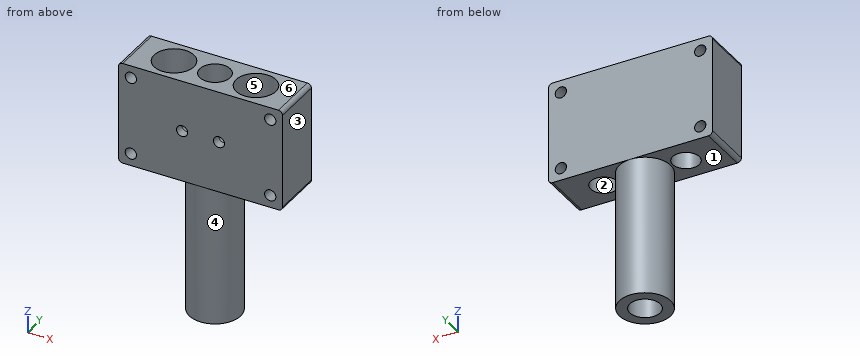
```python
from build123d import *
from OCP.BRepFilletAPI import BRepFilletAPI_MakeChamfer

# Parameters (mm, degrees)
SKETCH1_W            = 80
SKETCH1_H            = 50
BOSS_EXTRUDE1_DEPTH  = 25
M5_CLEARANCE_HOLE1_D = 5.5
SKETCH5_R            = 12.5
SKETCH5_R_2          = 6.985
BOSS_EXTRUDE2_DEPTH  = 68
SKETCH4_R            = 9.7
CUT_EXTRUDE2_DEPTH   = 29
SKETCH4_4_R          = 7.4
CUT_EXTRUDE3_DEPTH   = 128.078715763
SKETCH6_R            = 6.5
CUT_EXTRUDE4_DEPTH   = 101.727354775
BOSS_EXTRUDE3_START  = 1.3
SKETCH7_R            = 9.7
SKETCH7_R_2          = 9.5
BOSS_EXTRUDE3_DEPTH  = 1.3
CHAMFER2_SIZE        = 0.2
HOLE2_D              = 4.8
HOLE2_DEPTH          = 6
HOLE2_CBORE_D        = 5.4
HOLE2_CBORE_DEPTH    = 4
CHAMFER3_SIZE        = 4
CHAMFER3_SIZE_2      = 0.3
FILLET1_R            = 2


with BuildPart() as part:
    # Sketch1 → Boss-Extrude1 (new body)
    with BuildSketch(Plane(origin=(0, 0, 0), x_dir=(1, 0, 0), z_dir=(0, 1, 0))):
        Rectangle(SKETCH1_W, SKETCH1_H)
    extrude(amount=BOSS_EXTRUDE1_DEPTH)

    # M5 Clearance Hole1 (through all)
    with Locations(Plane(origin=(0, 25, 0), x_dir=(1, 0, 0), z_dir=(0, 1, 0))):
        with Locations((-34, 19), (34, 19), (34, -19), (-34, -19)):
            Hole(M5_CLEARANCE_HOLE1_D / 2)

    # Sketch5 → Boss-Extrude2 (add)
    with BuildSketch(Plane(origin=(0, 0, -25), x_dir=(-1, 0, 0), z_dir=(0, 0, -1))):
        with Locations(Location((0, 12.5, 0), (0, 0, 270))):
            Circle(SKETCH5_R)
        with Locations((0, 12.5)):
            Circle(SKETCH5_R_2, mode=Mode.SUBTRACT)
    extrude(amount=BOSS_EXTRUDE2_DEPTH)

    # Sketch4 → Cut-Extrude2 (cut)
    with BuildSketch(Plane.XY.offset(25)):
        with Locations((-20, 12.5)):
            Circle(SKETCH4_R)
        with Locations((20, 12.5)):
            Circle(SKETCH4_R)
    extrude(amount=-CUT_EXTRUDE2_DEPTH, mode=Mode.SUBTRACT)

    # Sketch4<4> → Cut-Extrude3 (cut, through all)
    with BuildSketch(Plane.XY.offset(25)):
        with Locations((0, 12.5)):
            Circle(SKETCH4_4_R)
    extrude(amount=-CUT_EXTRUDE3_DEPTH, mode=Mode.SUBTRACT)

    # Sketch6 → Cut-Extrude4 (cut, through all)
    with BuildSketch(Plane.XY.offset(-4)):
        with Locations((-20, 12.5)):
            Circle(SKETCH6_R)
        with Locations((20, 12.5)):
            Circle(SKETCH6_R)
    extrude(amount=-CUT_EXTRUDE4_DEPTH, mode=Mode.SUBTRACT)

    # Sketch7 → Boss-Extrude3 (add)
    # profile 1 of 2: a face of its own
    with BuildSketch(Plane.XY.offset(-0.5).offset(BOSS_EXTRUDE3_START)):
        with Locations((-20, 12.5)):
            Circle(SKETCH7_R)
        with Locations((-20, 12.5)):
            Circle(SKETCH7_R_2, mode=Mode.SUBTRACT)
    # profile 2 of 2: a face of its own
    with BuildSketch(Plane.XY.offset(-0.5).offset(BOSS_EXTRUDE3_START)):
        with Locations((20, 12.5)):
            Circle(SKETCH7_R)
        with Locations((20, 12.5)):
            Circle(SKETCH7_R_2, mode=Mode.SUBTRACT)
    extrude(amount=-BOSS_EXTRUDE3_DEPTH)

    # Chamfer2
    chamfer2_edges = [part.edges().sort_by_distance(p)[0] for p in [
        (-29.5, 12.5, -0.5),
        (-29.5, 12.5, 0.8),
        (10.5, 12.5, -0.5),
        (10.5, 12.5, 0.8),
    ]]
    chamfer(chamfer2_edges, length=CHAMFER2_SIZE - 0.0001)  # a hair under: the kernel refuses the full size

    # Hole2
    with Locations(Plane(origin=(0, 0, 0), x_dir=(-1, 0, 0), z_dir=(0, -1, 0))):
        with Locations((-9, 0), (9, 0)):
            CounterBoreHole(HOLE2_D / 2, HOLE2_CBORE_D / 2, HOLE2_CBORE_DEPTH, depth=HOLE2_DEPTH)

    # Chamfer3
    chamfer3_edges_1 = [part.edges().sort_by_distance(p)[0] for p in [
        (-6.3, 4, 0),
    ]]
    chamfer3_side_1 = [part.faces().sort_by_distance(p)[0] for p in [
        (-6.3, 3.994, 0),
    ]]
    chamfer3_edges_2 = [part.edges().sort_by_distance(p)[0] for p in [
        (11.7, 4, 0),
    ]]
    chamfer3_side_2 = [part.faces().sort_by_distance(p)[0] for p in [
        (11.7, 3.994, 0),
    ]]
    chamfer3 = BRepFilletAPI_MakeChamfer(part.part.solid().wrapped)
    for e in chamfer3_edges_1:
        chamfer3.Add(CHAMFER3_SIZE - 0.0001, CHAMFER3_SIZE_2 - 0.0001, e.wrapped, chamfer3_side_1[0].wrapped)
    for e in chamfer3_edges_2:
        chamfer3.Add(CHAMFER3_SIZE - 0.0001, CHAMFER3_SIZE_2 - 0.0001, e.wrapped, chamfer3_side_2[0].wrapped)
    add(Compound.cast(chamfer3.Shape()), mode=Mode.REPLACE)  # a hair under: the kernel refuses the full size

    # Fillet1
    fillet1_edges = [part.edges().sort_by_distance(p)[0] for p in [
        (40, 12.5, 25),
        (-40, 12.5, 25),
        (-40, 12.5, -25),
        (40, 12.5, -25),
    ]]
    fillet(fillet1_edges, radius=FILLET1_R)


solid = part.part
```
Input: part model. Units: mm. Frame: model coordinates. Face numbers are marked on the shaded views. A direction names the side the tool comes from. Give positions to 0.01 mm unless a question says otherwise; leave off trailing zeros. Write each loop counter-clockwise with the first axis right and the second up, starting at its lowest first coordinate (ties: lowest second). Pieces come first, ordered by that corner, then holes. Notation, with made-up numbers: (28.25, -26) - (44.25, -26) arc R26 cw to (44.25, 1) - close; hole circle Ø2 at (13, -38.5). An arc over 180 degrees is marked (long way). Write item = value, one per line. Start each with the question number.
1. Access query for the marked faces 4, 5 and 6. Directions: +Z, -Z, +X, -X, +Y, -Y. A direction counts if a zero-diameter tool reaches every point of the face in a straight line with its end or side. Return the directions, or none.
2. Mould query, pull axis X, two halves, no side actions, for the marked faces 1, 2 and 3. Classes: released by +X, released by -X, zero draft, split by the parting line, or undercut.
3. Section query A-A, the plane z = 19. Output: boundary loops of the cut face in (x, y), then the cut area to 3 significant figures.
4. First-contact query: pin 1 Ø4 at (x, y) = (27, 8) entering from -Z; pin 2 Ø2.5 at (x, z) = (8.5, 0.5) entering from -Y. Flat tips, straight axial feed; report the tip coordinate or a pass-through.
5. Section query D-D, the plane z = -71.5. Output: boundary loops of the cut face in (x, y).
6. Section query C-C, the plane x = -34. Output: boundary loops of the cut face in (y, z), then the cut area to 3 significant figures.
7. Ray query, L1, parallel to X at y = 0.05, z = 0; L2, parallel to Z at x = -34, y = 8.25; L3, parallel to Z at x = 32, y = 9.25. Return the intervals inside material, ascending.
Check sheet entries:
q1.face_4 = -Z
q1.face_5 = +Z
q1.face_6 = +Z, +X, -X, +Y, -Y
q2.face_1 = zero draft
q2.face_2 = undercut
q2.face_3 = released by +X
q3.outline = (-40, 0) - (-36.75, 0) - (-36.75, 25) - (-40, 25) - close; (-31.25, 0) - (31.25, 0) - (31.25, 25) - (-31.25, 25) - close; (36.75, 0) - (40, 0) - (40, 25) - (36.75, 25) - close; hole circle Ø19.4 at (-20, 12.5); hole circle Ø14.8 at (0, 12.5); hole circle Ø19.4 at (20, 12.5)
q3.area = 962 mm2
q4.pin_1 = -25
q4.pin_2 = 6
q5.outline = circle Ø25 at (0, 12.5); hole circle Ø14.8 at (0, 12.5)
q6.outline = (0, -25) - (25, -25) - (25, -21.75) - (0, -21.75) - close; (0, -16.25) - (25, -16.25) - (25, 16.25) - (0, 16.25) - close; (0, 21.75) - (25, 21.75) - (25, 25) - (0, 25) - close
q6.area = 975 mm2
q7.L1 = -40 to -11.7, -6.3 to 6.3, 11.7 to 40
q7.L2 = -25 to -21.75, -16.25 to 16.25, 21.75 to 25
q7.L3 = -25 to -20.89, -17.11 to 17.11, 20.89 to 25
